Verification items for the finished model (mm, model axes). Coordinates: 2 decimals unless noted, no trailing zeros. Order: outer loops, then holes, each group sorted by start corner. A loop starts at its lowest first (then second) coordinate and runs counter-clockwise, first axis right, second up. Notation, with made-up numbers: (27, 74) -> (35, 74) arc R27 cw to (35, 112) -> close; hole circle Ø4 at (39, 76). An arc over 180 degrees is marked (long way). Answer as CSV lines item,"result".
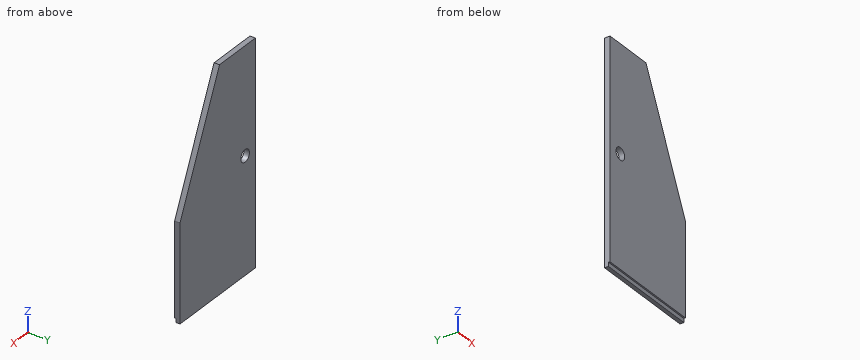
```python
from build123d import *

# Parameters (mm, degrees)
F0_R     = 3.6
F0_W     = 30
F0_H     = 45.876608
F0_W_2   = 63
F0_H_2   = 54.823392
F1_DEPTH = 3.2
F0_H_3   = 2.3
F2_DEPTH = 2.3


with BuildPart() as f1:
    # F0 (on Front) → F1 (new body)
    with BuildSketch(Plane.XZ):
        Polygon((-43.617142, 31.438855), (-43.617142, 4.438855), (19.382858, 4.438855), (-13.617142, 77.315463), (-13.617142, 31.438855), align=None)
        with Locations((-35.017142, 15.013501)):
            Circle(F0_R, mode=Mode.SUBTRACT)
        with Locations((-28.617142, 54.377159)):
            Rectangle(F0_W, F0_H)
        with Locations((-12.117142, -22.972841)):
            Rectangle(F0_W_2, F0_H_2)
    extrude(amount=F1_DEPTH)

    # F0 (on Front) → F2 (join)
    with BuildSketch(Plane.XZ):
        Polygon((-43.617142, 31.438855), (-43.617142, 4.438855), (19.382858, 4.438855), (-13.617142, 77.315463), (-13.617142, 31.438855), align=None)
        with Locations((-35.017142, 15.013501)):
            Circle(F0_R, mode=Mode.SUBTRACT)
        with Locations((-12.117142, -22.972841)):
            Rectangle(F0_W_2, F0_H_2)
        with Locations((-12.117142, -51.534537)):
            Rectangle(F0_W_2, F0_H_3)
        with Locations((-28.617142, 54.377159)):
            Rectangle(F0_W, F0_H)
    extrude(amount=F2_DEPTH)


solid = f1.part
```
Item 1: Thickness scan on line 1 (Z direction, x = -24, y = -2.35); line 2 (X direction, y = -1.5, z = 46); line 3 (Z direction, x = 14, y = -2.55). Record the ranges inside material, lowest first.
Answer list:
line 1,"-50.38 to 77.32"
line 2,"-43.62 to 0.56"
line 3,"-50.38 to 16.33"
Item 2: Section check A-A, the plane x = -33. Record the boundary of the cut face in (y, z).
Answer list:
outline,"(-3.2, -50.38) -> (-2.3, -50.38) -> (-2.3, -52.68) -> (0, -52.68) -> (0, 12.03) -> (-3.2, 12.03) -> close; (-3.2, 18) -> (0, 18) -> (0, 77.32) -> (-3.2, 77.32) -> close"
Item 3: Section check D-D, the plane z = 36. Record the boundary of the cut face in (x, y), plus the area to 3 significant figures.
Answer list:
outline,"(-43.62, -3.2) -> (5.09, -3.2) -> (5.09, 0) -> (-43.62, 0) -> close"
area,"156 mm2"
Item 4: Section check B-B, the plane y = -0.6. Record the boundary of the cut face in (x, z), plus the area to 3 significant figures.
Answer list:
outline,"(-43.62, -52.68) -> (19.38, -52.68) -> (19.38, 4.44) -> (-13.62, 77.32) -> (-43.62, 77.32) -> close; hole circle Ø7.2 at (-35.02, 15.01)"
area,"6,950 mm2"
Item 5: Section check C-C, the plane x = 3. Record the boundary of the cut face in (y, z).
Answer list:
outline,"(-3.2, -50.38) -> (-2.3, -50.38) -> (-2.3, -52.68) -> (0, -52.68) -> (0, 40.62) -> (-3.2, 40.62) -> close"
Item 6: Depth check by flat-ended pin: pin 1 Ø0.7 at (x, z) = (-26.5, -52) entering from -Y; pin 2 Ø6 at (x, z) = (-35.02, 15.01) entering from -Y; pin 3 Ø1.5 at (x, y) = (-11, -0.5) entering from +Z. Enter the tip coordinate at first touch or a pass-through.
Answer list:
pin 1,"y = -2.3"
pin 2,"through"
pin 3,"z = 73.19"
